from build123d import *

# Parameters (mm, degrees)
SKETCH1_R           = 28.5
SKETCH1_R_2         = 15
BOSS_EXTRUDE1_DEPTH = 38
SKETCH2_W           = 84
SKETCH2_H           = 57
BOSS_EXTRUDE2_DEPTH = 16
SKETCH3_R           = 8
BOSS_EXTRUDE3_DEPTH = 14
CUT_EXTRUDE1_START  = -38
CUT_EXTRUDE1_DEPTH  = 38
CUT_EXTRUDE2_START  = -38
SKETCH5_R           = 15
CUT_EXTRUDE2_DEPTH  = 38


with BuildPart() as part:
    # Sketch1 → Boss-Extrude1 (new body)
    with BuildSketch(Plane(origin=(0, 0, 0), x_dir=(1, 0, 0), z_dir=(0, 1, 0))):
        with Locations(Location((0, 0, 0), (0, 0, 270))):
            Circle(SKETCH1_R)
        with Locations(Location((0, 0, 0), (0, 0, 270))):
            Circle(SKETCH1_R_2, mode=Mode.SUBTRACT)
    extrude(amount=BOSS_EXTRUDE1_DEPTH)

    # Sketch2 → Boss-Extrude2 (add)
    with BuildSketch(Plane.XZ):
        Rectangle(SKETCH2_W, SKETCH2_H)
    extrude(amount=BOSS_EXTRUDE2_DEPTH)

    # Sketch3 → Boss-Extrude3 (add)
    with BuildSketch(Plane(origin=(42, 0, 0), x_dir=(0, 0, -1), z_dir=(1, 0, 0))):
        with BuildLine():
            Line((-28.5, -16), (-18.629891095, -41.275105345))
            ThreePointArc((-18.629891095, -41.275105345), (0, -54), (18.629891095, -41.275105345))
            Line((18.629891095, -41.275105345), (28.5, -16))
            Line((28.5, -16), (-28.5, -16))
        make_face()
        with Locations((0, -34)):
            Circle(SKETCH3_R, mode=Mode.SUBTRACT)
    boss_extrude3 = extrude(amount=-BOSS_EXTRUDE3_DEPTH)

    # Mirror1: Boss-Extrude3 across plane
    add(boss_extrude3.mirror(Plane(origin=(0, 0, 0), x_dir=(0, 0, 1), z_dir=(1, 0, 0))))

    # Sketch4 → Cut-Extrude1 (cut)
    with BuildSketch(Plane(origin=(0, 38, 0), x_dir=(1, 0, 0), z_dir=(0, 1, 0)).offset(CUT_EXTRUDE1_START)):
        with BuildLine():
            Line((-4, -14.456832295), (-4, -17.456832295))
            Line((-4, -17.456832295), (4, -17.456832295))
            Line((4, -17.456832295), (4, -14.456832295))
            ThreePointArc((4, -14.456832295), (0, -15), (-4, -14.456832295))
        make_face()
    extrude(amount=CUT_EXTRUDE1_DEPTH, mode=Mode.SUBTRACT)

    # Sketch5 → Cut-Extrude2 (cut)
    with BuildSketch(Plane(origin=(0, 0, 0), x_dir=(1, 0, 0), z_dir=(0, 1, 0)).offset(CUT_EXTRUDE2_START)):
        with Locations(Location((0, 0, 0), (0, 0, 90))):
            Circle(SKETCH5_R)
    extrude(amount=CUT_EXTRUDE2_DEPTH, mode=Mode.SUBTRACT)


solid = part.part
Work out the finished part from the listing and answer in its coordinate system (mm). A direction names the side the tool comes from. Round coordinates to 2 decimals unless told otherwise and drop trailing zeros. Write each loop counter-clockwise with the first axis right and the second up, starting at its lowest first coordinate (ties: lowest second). Pieces come first, ordered by that corner, then holes.
1) A cutting plane is placed at D-D (y = -11.5). Give the vertices of the cut face in (x, z), plus the area to 3 significant figures.
2) A tool of negligible diameter and unlimited length cuts with its end or side. For faces 5 (the flat face through (-13, -16, 13)), 6 (the flat face through (-31, 0, 0)), 7 (the cylindrical face through (-35, -54, 0)), 8 (the flat face through (0, 19, 17.457)), from which of +Z, -Z, +X, -X, +Y, -Y can it reach the whole face along a straight path? Write none if from no direction.
3) Given pin 1 Ø1.5 at (x, z) = (1, 16.5) entering from +Y; pin 2 Ø1 at (y, z) = (24.5, -5.5) entering from +X; pin 3 Ø10 at (x, z) = (2.5, -11.5) entering from -Y, each flat-ended and moving along its own axis, determine where each tip first touches the part or whether it passes through.
4) Straight lines are drawn through the part: line 1 (X direction, y = -19.5, z = -6); line 2 (Y direction, x = -35, z = 0); line 3 (Y direction, x = 14, z = -10). For each, find the intervals that lie inside material, in ascending order.
5) A cutting plane is placed at A-A (z = 12). Give the vertices of the cut face in (x, y), plus the area to 3 significant figures.
6) A cutting plane is placed at B-B (x = 32.5). Give the vertices of the cut face in (y, z), plus the area to 3 significant figures.
7) A cutting plane is placed at C-C (z = 0). Give the vertices of the cut face in (x, y).
8) The mould has two halves that part along Z. Classify faces 1 (the cylindrical face through (-35.098, -26.068, 1.041)), 2 (the flat face through (42, -21, 0)), 3 (the flat face through (-35.098, -28.461, 23.634)), 4 (the cylindrical face through (-27.82, 18.73, -6.18)): pulls with the +Z half, pulls with the -Z half, needs draft (parallel to the pull), parting line crosses it, or undercut.
Completed:
1. outline: (-42, -28.5) - (42, -28.5) - (42, 28.5) - (-42, 28.5) - close; hole circle Ø30 at (0, 0)
1. area: 4,080 mm2
2. face 5: +Z, -Z, -Y
2. face 6: -X, +Y
2. face 7: +X, -X, -Y
2. face 8: +Y
3. pin 1: stops at y = 0
3. pin 2: stops at x = 28.06
3. pin 3: stops at y = -16
4. line 1: x = -42 to -28, 28 to 42
4. line 2: y = -54 to -42, -26 to 0
4. line 3: y = -16 to 38
5. outline: (-42, -50) - (-28, -50) - (-28, -16) - (-9, -16) - (-9, 38) - (-25.85, 38) - (-25.85, 0) - (-42, 0) - close; (9, -16) - (28, -16) - (28, -50) - (42, -50) - (42, 0) - (25.85, 0) - (25.85, 38) - (9, 38) - close
5. area: 3,290 mm2
6. outline: (-41.28, -18.63) - (-16, -28.5) - (0, -28.5) - (0, 28.5) - (-16, 28.5) - (-41.28, 18.63) arc R20 ccw to start; hole circle Ø16 at (-34, 0)
6. area: 2,250 mm2
7. outline: (-42, -54) - (-28, -54) - (-28, -42) - (-42, -42) - close; (-42, -26) - (-28, -26) - (-28, -16) - (-15, -16) - (-15, 38) - (-28.5, 38) - (-28.5, 0) - (-42, 0) - close; (15, -16) - (28, -16) - (28, -26) - (42, -26) - (42, 0) - (28.5, 0) - (28.5, 38) - (15, 38) - close; (28, -54) - (42, -54) - (42, -42) - (28, -42) - close
8. face 1: undercut
8. face 2: needs draft
8. face 3: pulls with the +Z half
8. face 4: parting line crosses it
